Autodesk Inventor part; units mm, degrees
ref_plane "YZ Plane" through (0, 0, 0) normal (1, 0, 0) x (0, 1, 0)
ref_plane "XZ Plane" through (0, 0, 0) normal (0, 1, 0) x (-1, 0, 0)
ref_plane "XY Plane" through (0, 0, 0) normal (0, 0, 1) x (1, 0, 0)
sketch "草圖1" plane through (0, 0, 0) normal (0, 0, 1) x (1, 0, 0)
  line L0 (-7.5, 10) -> (7.5, 10)
  line L1 (7.5, 10) -> (7.5, -10)
  line L2 (7.5, -10) -> (-7.5, -10)
  line L3 (-7.5, -10) -> (-7.5, 10)
  line L4 (-7.5, 10) -> (7.5, -10) construction
  line L5 (7.5, 10) -> (-7.5, -10) construction
  point P0 (0, 0)
  dimension "d0" = 15
  dimension "d1" = 20
extrude "擠出1" add sketch "草圖1" along normal blind 15
sketch "草圖2" plane through (-7.5, 10, 0) normal (0, 1, 0) x (1, 0, 0)
  line L0 (0, 0) -> (0, -15)
  line L1 (0, -7.5) -> (15, -7.5)
  line L2 (15, 0) -> (15, -15)
  point P0 (7.5, 0)
sketch "草圖3" plane through (7.5, -10, 0) normal (1, 0, 0) x (0, 0, -1)
  line L0 (0, 0) -> (0, 20)
  line L1 (0, 20) -> (-15, 20)
  line L2 (-15, 0) -> (-15, 20)
  line L3 (-15, 20) -> (0, 20)
  line L4 (-7.5, 27.5) -> (-7.3, 27.5)
  line L5 (-7.5, 27.5) -> (-7.7, 27.5)
  line L6 (-7.3, 27.5) -> (0, 20)
  line L7 (-7.7, 27.5) -> (-15.0055, 20)
  line L8 (-7.7, 27.5) -> (-7.7, 30.5)
  line L9 (-7.7, 30.5) -> (-7.3, 30.5)
  line L10 (-7.3, 30.5) -> (-7.3, 27.5)
  line L11 (-15.0055, 20) -> (0, 20)
  point P0 (0, 10)
  point P1 (-7.5, 20)
  dimension "d4" = 7.5
  dimension "d5" = 0.2
  dimension "d6" = 3
extrude "擠出3" add sketch "草圖3" against normal blind 15
sketch "草圖4" plane through (-7.5, -10, 0) normal (-1, 0, 0) x (0, 0, 1)
  line L0 (0, 20) -> (7.3, 27.5)
  line L1 (0, 20) -> (15.0055, 20)
  line L2 (15.0055, 20) -> (7.5027, 20)
  line L3 (7.3, 30.5) -> (7.3, 27.5)
  line L4 (7.5027, 26.3355) -> (0, 20)
  line L5 (7.5027, 26.3355) -> (15.0055, 20)
  point P0 (0, 10)
extrude "擠出4" cut sketch "草圖4" against normal blind 5
properties part number "牛奶瓶"
The listing builds one solid part. Answer for the finished solid, in the listing's coordinates (mm). A direction names the side the tool comes from. Coordinates: 2 decimals unless noted, no trailing zeros. Loops run counter-clockwise (first coordinate to the right, second up) from the corner with the lowest first, then second, coordinate; pieces in that order, holes last. Notation, with made-up numbers: (-6, 55) -> (1, 55) arc R27 cw to (1, 75) -> close; hole circle Ø4 at (29.5, -5). An arc over 180 degrees is marked (long way). Return JSON: item names as keys, results as strings. Group by question number.
(1) Which of the six approach directions +Z, -Z, +X, -X, +Y, -Y give full straight-line access (tool end or side, diameter ignored) to faces 4 (the flat face through (0, 0, 0)), 5 (the flat face through (0, 19, 7.3)), 6 (the flat face through (-5, 10, 7)), 7 (the flat face through (0, 19, 7.7))?
(2) Find the intervals of material crossed by probe 1 along Z at (x, y) = (3.5, -3); probe 2 along Y at (x, z) = (-3.5, 8.25); probe 3 along Y at (x, z) = (-4, 2.5), in increasing order. Write a range as from..to.
(3) Given pin 1 Ø4.5 at (x, y) = (-0.5, 3) entering from +Z; pin 2 Ø0.9 at (x, y) = (-1.5, 19.5) entering from -Z; pin 3 Ø3.5 at (x, y) = (-0.5, 18.5) entering from +Z, each flat-ended and moving along its own axis, determine where each tip first touches the part or whether it passes through.
(4) A cutting plane is placed at C-C on y = 12. Write down the section's boundary in (x, z).
(5) Determine the mould class of faces 1 (the flat face through (-7.5, 15.61, 6.36)), 2 (the flat face through (-2.5, 13, 7)), 3 (the flat face through (0, -10, 7)) for opening direction Y: released by +Y, released by -Y, zero draft, split by the parting line, or undercut.
(6) A cutting plane is placed at B-B on z = 12.25. Write down the section's boundary in (x, y).
The answers:
{
 "1": {"face 4": "-Z, +X, -X, +Y, -Y", "face 5": "-Z, +X, -X, +Y", "face 6": "-X", "face 7": "+Z, +X, -X, +Y"},
 "2": {"probe 1": "z = 0..15", "probe 2": "y = -10..10, 15.7..16.94", "probe 3": "y = -10..10, 12.11..12.57"},
 "3": {"pin 1": "stops at z = 15", "pin 2": "stops at z = 7.3", "pin 3": "stops at z = 8.43"},
 "4": {"outline": "(-7.5, 1.95) -> (7.5, 1.95) -> (7.5, 13.06) -> (-7.5, 13.06) -> (-7.5, 12.64) -> (-2.5, 12.64) -> (-2.5, 2.37) -> (-7.5, 2.37) -> close"},
 "5": {"face 1": "zero draft", "face 2": "undercut", "face 3": "released by -Y"},
 "6": {"outline": "(-7.5, -10) -> (7.5, -10) -> (7.5, 12.83) -> (-7.5, 12.83) -> (-7.5, 12.33) -> (-2.5, 12.33) -> (-2.5, 10) -> (-7.5, 10) -> close"}
}
